Verification items for the finished model (mm, model axes). Face numbers are marked on the shaded views. A direction names the side the tool comes from. Round coordinates to 2 decimals unless told otherwise and drop trailing zeros. Write each loop counter-clockwise with the first axis right and the second up, starting at its lowest first coordinate (ties: lowest second). Pieces come first, ordered by that corner, then holes. Notation, with made-up numbers: M -12.75,-12 L 43.25,-12 A19 ccw 43.25,18 Z; hole C -38,-3.75 d11. An arc over 180 degrees is marked long. One line per question, with ' | ' between items.
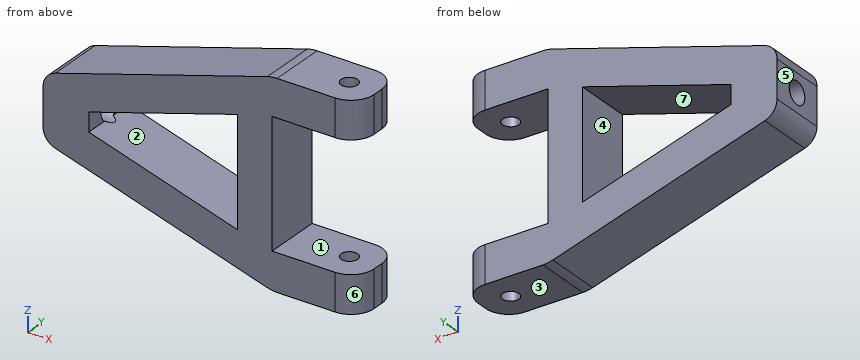
from build123d import *

# Parameters (mm, degrees)
SKETCH1_W           = 55
SKETCH1_H           = 35
BOSS_EXTRUDE1_DEPTH = 10
CUT_EXTRUDE6_DEPTH  = 66.954529791
SKETCH12_R          = 1.45
CUT_EXTRUDE8_DEPTH  = 66.954529791
SKETCH13_R          = 1.95
CUT_EXTRUDE9_DEPTH  = 11
SKETCH2_W           = 22
SKETCH2_H           = 10
CUT_EXTRUDE10_DEPTH = 15
FILLET4_R           = 4
FILLET5_R           = 3
FILLET6_R           = 6
CUT_EXTRUDE11_DEPTH = 66.954529791


with BuildPart() as part:
    # Sketch1 → Boss-Extrude1 (new body)
    with BuildSketch(Plane(origin=(0, 0, 0), x_dir=(1, 0, 0), z_dir=(0, 1, 0))):
        with Locations((27.5, -17.5)):
            Rectangle(SKETCH1_W, SKETCH1_H)
    extrude(amount=BOSS_EXTRUDE1_DEPTH)

    # Sketch9 → Cut-Extrude6 (cut, through all)
    with BuildSketch(Plane(origin=(0, 0, 0), x_dir=(-1, 0, 0), z_dir=(0, -1, 0))):
        Polygon((0, -12), (-40, 0), (0, 0), align=None)
        Polygon((0, -23), (-40, -35), (0, -35), align=None)
    extrude(amount=-CUT_EXTRUDE6_DEPTH, mode=Mode.SUBTRACT)

    # Sketch12 → Cut-Extrude8 (cut, through all)
    with BuildSketch(Plane.XY.offset(35)):
        with Locations((50, 5)):
            Circle(SKETCH12_R)
    extrude(amount=-CUT_EXTRUDE8_DEPTH, mode=Mode.SUBTRACT)

    # Sketch13 → Cut-Extrude9 (cut)
    with BuildSketch(Plane.ZY):
        with Locations((17.5, 5)):
            Circle(SKETCH13_R)
    extrude(amount=-CUT_EXTRUDE9_DEPTH, mode=Mode.SUBTRACT)

    # Sketch2 → Cut-Extrude10 (cut)
    with BuildSketch(Plane(origin=(55, 0, 0), x_dir=(0, 0, -1), z_dir=(1, 0, 0))):
        with Locations((-17.5, 5)):
            Rectangle(SKETCH2_W, SKETCH2_H)
    extrude(amount=-CUT_EXTRUDE10_DEPTH, mode=Mode.SUBTRACT)

    # Fillet4
    fillet4_edges = [part.edges().sort_by_distance(p)[0] for p in [
        (55, 10, 31.75),
        (55, 0, 3.25),
        (55, 10, 3.25),
        (55, 0, 31.75),
    ]]
    fillet(fillet4_edges, radius=FILLET4_R)

    # Fillet5
    fillet5_edges = [part.edges().sort_by_distance(p)[0] for p in [
        (0, 5, 12),
        (0, 5, 23),
    ]]
    fillet(fillet5_edges, radius=FILLET5_R)

    # Fillet6
    fillet6_edges = [part.edges().sort_by_distance(p)[0] for p in [
        (40, 5, 0),
        (40, 5, 35),
    ]]
    fillet(fillet6_edges, radius=FILLET6_R)

    # Sketch15 → Cut-Extrude11 (cut, through all)
    with BuildSketch(Plane(origin=(0, 0, 0), x_dir=(-1, 0, 0), z_dir=(0, -1, 0))):
        Polygon((-34, -26.935816095), (-8, -19.135816095), (-8, -15.864183905), (-34, -8.064183905), align=None)
    extrude(amount=-CUT_EXTRUDE11_DEPTH, mode=Mode.SUBTRACT)


solid = part.part
1. Tool access check on the marked faces 1, 2 and 3. Record the directions out of +Z, -Z, +X, -X, +Y, -Y that give a thin tool (end or side, any length) a straight path to the whole face; none if there is none.
Results:
face 1: +X, +Y, -Y | face 2: +Y, -Y | face 3: -Z, +X, -X, +Y, -Y
2. Go/stop test with flat-tipped pins: P1, Ø1, axis at x = 7.5, y = 6, coming from the -Z side; P2, Ø1.5, axis at y = 5, z = 22, coming from the +X side; P3, Ø1, axis at x = 24, y = 7, coming from the -Z side. Record where each tip stops, or that it passes through.
Results:
P1: stops at z = 9.6 | P2: stops at x = 40 | P3: stops at z = 4.65
3. Section check D-D, the plane z = 32. Record the cut outline in (x, y), then the cut area to 3 significant figures.
Results:
outline: M 30,0 L 51,0 A4 ccw 55,4 L 55,6 A4 ccw 51,10 L 30,10 Z; hole C 50,5 d2.9 | area: 237 mm2
4. Section check B-B, the plane z = 17.5. Record the cut outline in (x, y).
Results:
outline: M 0,0 L 8,0 L 8,3.05 L 0,3.05 Z; M 0,6.95 L 8,6.95 L 8,10 L 0,10 Z; M 34,0 L 40,0 L 40,10 L 34,10 Z
5. Section check C-C, the plane x = 47.5. Record the cut outline in (y, z).
Results:
outline: M 0,0 L 10,0 L 10,6.5 L 0,6.5 Z; M 0,28.5 L 10,28.5 L 10,35 L 0,35 Z
6. Thickness scan on line 1 (Y direction, x = 50, z = 4); line 2 (Z direction, x = 43.5, y = 2); line 3 (Y direction, x = 5, z = 17.5). Record the ranges inside material, lowest first.
Results:
line 1: y = 0 to 3.55, 6.45 to 10 | line 2: z = 0 to 6.5, 28.5 to 35 | line 3: y = 0 to 3.05, 6.95 to 10
7. Mould release check, pull along X, two halves, no side actions. Record for the marked faces 4, 5, 6 and 7: pulls with the +X half, pulls with the -X half, needs draft (parallel to the pull), parting line crosses it, or undercut.
Results:
face 4: undercut | face 5: pulls with the -X half | face 6: pulls with the +X half | face 7: undercut
8. Section check A-A, the plane y = 5. Record the cut outline in (x, z), then the cut area to 3 significant figures.
Results:
outline: M 0,14.23 A3 ccw 2.14,11.36 L 39.16,0.25 A6 ccw 40.88,0 L 48.55,0 L 48.55,6.5 L 40,6.5 L 40,28.5 L 48.55,28.5 L 48.55,35 L 40.88,35 A6 ccw 39.16,34.75 L 2.14,23.64 A3 ccw 0,20.77 L 0,19.45 L 9.05,19.45 L 34,26.94 L 34,8.06 L 9.05,15.55 L 0,15.55 Z; M 51.45,0 L 55,0 L 55,6.5 L 51.45,6.5 Z; M 51.45,28.5 L 55,28.5 L 55,35 L 51.45,35 Z | area: 756 mm2
